from build123d import *

# Parameters (mm, degrees)
PAD_DEPTH   = 37.5
FILLET_R    = 2
FILLET001_R = 0.4


with BuildPart() as part:
    # Sketch → Pad (new body)
    with BuildSketch(Plane.XY):
        with BuildLine():
            Line((0, 0), (4.5, 0))
            Line((4.5, 0), (4.5, 3))
            Line((4.5, 3), (3.3, 3))
            ThreePointArc((2.5, 3.8), (1.934315, 2.434315), (3.3, 3))
            Line((2.5, 14.8), (2.5, 3.8))
            ThreePointArc((3.3, 15.6), (1.934315, 16.165685), (2.5, 14.8))
            Line((6.325, 15.6), (3.3, 15.6))
            Line((6.325, 15.6), (6.325, 23.6))
            Line((6.325, 23.6), (28.825, 23.6))
            Line((28.825, 23.6), (28.825, 15.6))
            Line((28.825, 15.6), (31.85, 15.6))
            ThreePointArc((32.65, 14.8), (33.215685, 16.165685), (31.85, 15.6))
            Line((32.65, 14.8), (32.65, 3.8))
            ThreePointArc((31.85, 3), (33.215685, 2.434315), (32.65, 3.8))
            Line((30.65, 3), (31.85, 3))
            Line((30.65, 3), (30.65, 0))
            Line((30.65, 0), (35.15, 0))
            Line((35.15, 0), (35.15, 26.6))
            Line((35.15, 26.6), (0, 26.6))
            Line((0, 26.6), (0, 0))
        make_face()
    extrude(amount=PAD_DEPTH)

    # Fillet
    fillet_edges = [part.edges().sort_by_distance(p)[0] for p in [
        (0, 26.6, 18.75),
        (0, 0, 18.75),
        (4.5, 0, 18.75),
        (30.65, 0, 18.75),
        (35.15, 0, 18.75),
        (35.15, 26.6, 18.75),
    ]]
    fillet(fillet_edges, radius=FILLET_R)

    # Fillet001
    fillet001_edges = [part.edges().sort_by_distance(p)[0] for p in [
        (6.325, 15.6, 18.75),
        (6.325, 23.6, 18.75),
        (28.825, 23.6, 18.75),
        (28.825, 15.6, 18.75),
        (4.5, 3, 18.75),
        (30.65, 3, 18.75),
        (3.3, 15.6, 18.75),
        (31.85, 15.6, 18.75),
        (2.5, 14.8, 18.75),
        (32.65, 14.8, 18.75),
        (3.3, 3, 18.75),
        (31.85, 3, 18.75),
        (32.65, 3.8, 18.75),
        (2.5, 3.8, 18.75),
    ]]
    fillet(fillet001_edges, radius=FILLET001_R)


solid = part.part
Here's how the part is built. I have some questions about the finished solid (model axes, mm). A direction names the side the tool comes from. Round coordinates to 2 decimals unless told otherwise and drop trailing zeros. Loops run counter-clockwise (first coordinate to the right, second up) from the corner with the lowest first, then second, coordinate; pieces in that order, holes last. Notation, with made-up numbers: M 52,71.25 L 56,71.25 A17 cw 56,87.25 Z; hole C -22,0.25 d11. An arc over 180 degrees is marked long. Write each question's results on one line, items separated by ' | '. Start each with the question number.
(1) I want a section at C-C (x = 18). Please give me the cut outline in (y, z).
(2) If I drill on probe 1 along X at (y, z) = (20.25, 29) (3 decimals); probe 2 along X at (y, z) = (5, 3.5); probe 3 along Y at (x, z) = (23, 14), over which ranges is the centre line in solid material (lowest first)? Write a range as from..to.
(3) Will these pins go through, and if not, where does the flat tip stop? P1, Ø2.5, axis at x = 30.5, z = 14, coming from the -Y side; P2, Ø11, axis at x = 23, z = 23, coming from the -Y side; P3, Ø3, axis at x = 14.5, y = 23.5, coming from the -Z side; P4, Ø12, axis at x = 23.5, z = 11, coming from the -Y side.
(4) I want a section at B-B (y = 22). Please give me the cut outline in (x, z) (3 decimals).
(5) Thinking about a two-plate mould opening in Y: for faces 4 (the flat face through (17, 25, 37.5)), 5 (the cylindrical face through (0.6, 0.57, 19.01)), 6 (the cylindrical face through (1.92, 2.45, 18.49)), 7 (the cylindrical face through (0.6, 26.03, 19.01)), which applies, pulls with the +Y half, pulls with the -Y half, needs draft (parallel to the pull), parting line crosses it, or undercut?
(6) I want a section at A-A (y = 7.25). Please give me the cut outline in (x, z), then the cut area to 4 significant figures.
(7) On a 3-axis mill with a long thin cutter (end or side, diameter ignored), from which of +Z, -Z, +X, -X, +Y, -Y can I reach the whole of each face in a straight line? I mean faces 1 (the flat face through (6.325, 20, 18)), 2 (the flat face through (30, 15.6, 18)), 3 (the flat face through (17, 25, 0)). Say none if no direction works.
Solved:
1) outline: M 23.6,0 L 26.6,0 L 26.6,37.5 L 23.6,37.5 Z
2) probe 1: x = 0..6.325, 28.825..35.15 | probe 2: x = 0..2.5, 32.65..35.15 | probe 3: y = 23.6..26.6
3) P1: stops at y = 0.21 | P2: stops at y = 23.59 | P3: stops at z = 0 | P4: stops at y = 15.6
4) outline: M 0,0 L 6.325,0 L 6.325,37.5 L 0,37.5 Z; M 28.825,0 L 35.15,0 L 35.15,37.5 L 28.825,37.5 Z
5) face 4: needs draft | face 5: pulls with the -Y half | face 6: undercut | face 7: pulls with the +Y half
6) outline: M 0,0 L 2.5,0 L 2.5,37.5 L 0,37.5 Z; M 32.65,0 L 35.15,0 L 35.15,37.5 L 32.65,37.5 Z | area: 187.5 mm²
7) face 1: +Z, -Z, -Y | face 2: +Z, -Z | face 3: -Z, +X, -X, +Y, -Y
